Read the model definition and answer for the solid it produces. Units are mm, in the model's axes. Give positions to 0.01 mm unless a question says otherwise; leave off trailing zeros. Write each loop counter-clockwise with the first axis right and the second up, starting at its lowest first coordinate (ties: lowest second). Pieces come first, ordered by that corner, then holes. Notation, with made-up numbers: (69.25, 40) - (76.25, 40) arc R29 ccw to (76.25, 64) - close; hole circle Ø9 at (-30, 26.5). An arc over 180 degrees is marked (long way). Answer as CSV lines item,"result".
```python
from build123d import *

# Parameters (mm, degrees)
F1_DEPTH = 1.27
F2_SIZE2 = 0.635
F2_SIZE  = 5.08
F3_SIZE2 = 5.07999
F3_SIZE  = 0.63499


# Not quite as in the source:
# - a fillet or chamfer is up to 0.001 mm smaller than in the source, because OpenCascade refuses the exact size


with BuildPart() as f1:
    # F0 (on Top) → F1 (new body)
    with BuildSketch(Plane.XY):
        with BuildLine():
            Line((-36.8330654015, 25.4), (-36.8330654015, 0))
            Line((-36.8330654015, 0), (-31.7530654015, 0))
            Line((-31.7530654015, 0), (-31.7530654015, 25.4))
            Line((-31.7530654015, 25.4), (-31.7530654015, 38.1))
            ThreePointArc((-31.7530654015, 38.1), (-23.9034396028, 58.5352834398), (-36.8330654015, 76.2))
            Line((-36.8330654015, 76.2), (-36.8330654015, 25.4))
        make_face()
    extrude(amount=F1_DEPTH)

    # F2
    f2_edges = [f1.edges().sort_by_distance(p)[0] for p in [
        (-23.90344, 58.535283, 1.27),
    ]]
    f2_side = f1.faces().sort_by_distance((-32.33426, 43.519124, 1.27))[0]
    chamfer(f2_edges, length=F2_SIZE, length2=F2_SIZE2, reference=f2_side)

    # F3 (size 0.635 and 5.08 in the source; OpenCascade refuses exactly that, so slightly less here)
    f3_edges = [f1.edges().sort_by_distance(p)[0] for p in [
        (-23.90344, 58.535283, 0),
    ]]
    f3_side = f1.faces().sort_by_distance((-23.90344, 58.535283, 0.3175))[0]
    chamfer(f3_edges, length=F3_SIZE, length2=F3_SIZE2, reference=f3_side)


solid = f1.part
```
(1) A cutting plane is placed at A-A (y = 5.5). Write down the section's boundary in (x, z).
Worked out:
outline,"(-36.83, 0) - (-31.75, 0) - (-31.75, 1.27) - (-36.83, 1.27) - close"
(2) This flat-tipped pin is pushed along its axis until it touches: P1, Ø5, axis at x = -29, y = 67.5, coming from the +Z side. Where does it stop, or does it pass through?
Worked out:
P1,"stops at z = 1.15"
(3) Find the intervals of material crossed by L1, parallel to X at y = 7.5, z = 0.1; L2, parallel to Z at x = -26, y = 48.5, in increasing order.
Worked out:
L1,"x = -36.83 to -31.75"
L2,"z = 0.49 to 0.78"
(4) A cutting plane is placed at B-B (z = 1.05). Write down the section's boundary in (x, y).
Worked out:
outline,"(-36.83, 0) - (-31.75, 0) - (-31.75, 42.77) arc R19.54 ccw to (-36.83, 72.46) - close"
